from build123d import *

# Parameters (mm, degrees)
STOCK_BOX_1_START         = 83.223281248
STOCK_BOX_1_OUTLINE_W     = 122
STOCK_BOX_1_OUTLINE_H     = 102
STOCK_BOX_1_DEPTH         = 5
STOCK_BOX_1_START_2       = 80.223281248
STOCK_BOX_1_2_OUTLINE_W   = 118
STOCK_BOX_1_2_OUTLINE_H   = 98
STOCK_BOX_1_2_OUTLINE_W_2 = 114
STOCK_BOX_1_2_OUTLINE_H_2 = 94
STOCK_BOX_1_2_DEPTH       = 3
CUT_EXTRUDE2_REACH        = 168.26
SKETCH2_W                 = 19
SKETCH2_H                 = 3
SKETCH2_W_2               = 11
SKETCH3_W                 = 122
SKETCH3_H                 = 102
BOSS_EXTRUDE1_DEPTH       = 3
SKETCH4_W                 = 122
SKETCH4_H                 = 102
CUT_EXTRUDE3_DEPTH        = 3


# Read off the part's stored shape, not the designer's step: Stock-Box-1
with BuildPart() as part:
    # Stock-Box-1 outline → Stock-Box-1 (new body)
    with BuildSketch(Plane(origin=(0, 0, 0), x_dir=(1, 0, 0), z_dir=(0, 1, 0)).offset(STOCK_BOX_1_START)):
        with Locations((6.476673428, -22.886409736)):
            Rectangle(STOCK_BOX_1_OUTLINE_W, STOCK_BOX_1_OUTLINE_H)
    extrude(amount=STOCK_BOX_1_DEPTH)

    # Stock-Box-1 2 outline → Stock-Box-1 2 (add)
    with BuildSketch(Plane(origin=(0, 0, 0), x_dir=(1, 0, 0), z_dir=(0, 1, 0)).offset(STOCK_BOX_1_START_2)):
        with Locations((6.476673428, -22.886409736)):
            Rectangle(STOCK_BOX_1_2_OUTLINE_W, STOCK_BOX_1_2_OUTLINE_H)
        with Locations((6.476673428, -22.886409736)):
            Rectangle(STOCK_BOX_1_2_OUTLINE_W_2, STOCK_BOX_1_2_OUTLINE_H_2, mode=Mode.SUBTRACT)
    extrude(amount=STOCK_BOX_1_2_DEPTH)

    # Sketch2 → Cut-Extrude2 (cut, up to next)
    with BuildSketch(Plane.ZY.offset(52.523326572), mode=Mode.PRIVATE) as cut_extrude2_sk1:
        with Locations((-3.613590264, 81.723281248)):
            Rectangle(SKETCH2_W, SKETCH2_H)
    cut_extrude2_tool1 = extrude(cut_extrude2_sk1.sketch, amount=-CUT_EXTRUDE2_REACH, mode=Mode.PRIVATE) & part.part
    # Sketch2 → Cut-Extrude2 (cut, up to next)
    with BuildSketch(Plane.ZY.offset(52.523326572), mode=Mode.PRIVATE) as cut_extrude2_sk2:
        with Locations((21.386409736, 81.723281248)):
            Rectangle(SKETCH2_W_2, SKETCH2_H)
    cut_extrude2_tool2 = extrude(cut_extrude2_sk2.sketch, amount=-CUT_EXTRUDE2_REACH, mode=Mode.PRIVATE) & part.part
    add(cut_extrude2_tool1.solids().sort_by_distance((-52.523327, 81.723281, -3.61359))[0], mode=Mode.SUBTRACT)
    add(cut_extrude2_tool2.solids().sort_by_distance((-52.523327, 81.723281, 21.38641))[0], mode=Mode.SUBTRACT)

    # Sketch3 → Boss-Extrude1 (add)
    with BuildSketch(Plane(origin=(0, 88.223281248, 0), x_dir=(1, 0, 0), z_dir=(0, 1, 0))):
        with Locations((6.476673428, -22.886409736)):
            Rectangle(SKETCH3_W, SKETCH3_H)
    extrude(amount=-BOSS_EXTRUDE1_DEPTH)

    # Sketch4 → Cut-Extrude3 (cut)
    with BuildSketch(Plane(origin=(0, 88.223281248, 0), x_dir=(1, 0, 0), z_dir=(0, 1, 0))):
        with Locations((6.476673428, -22.886409736)):
            Rectangle(SKETCH4_W, SKETCH4_H)
    extrude(amount=-CUT_EXTRUDE3_DEPTH, mode=Mode.SUBTRACT)


solid = part.part
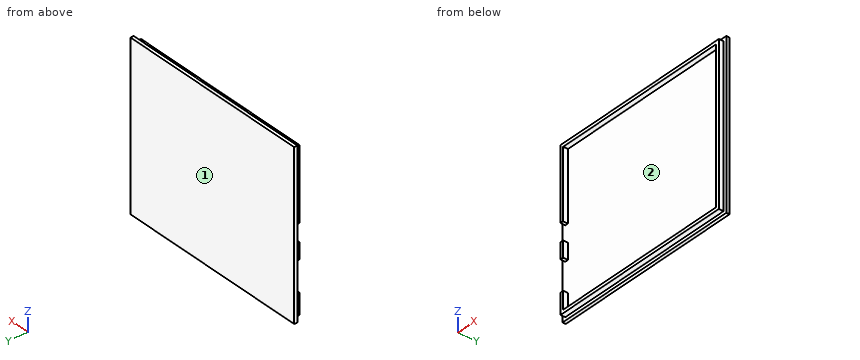
Verification items for the finished model (mm, model axes). Face numbers are marked on the shaded views. Coordinates: 2 decimals unless noted, no trailing zeros. Loops run counter-clockwise (first coordinate to the right, second up) from the corner with the lowest first, then second, coordinate; pieces in that order, holes last. Notation, with made-up numbers: (68, -6.5) -> (107, -6.5) arc R11 ccw to (107, 14.5) -> close; hole circle Ø3 at (37.25, 61). An arc over 180 degrees is marked (long way). Answer as a JSON object with one key per item and string values. Group by question number.
Item 1: Scan lines: probe 1 along X at (y, z) = (82.05, 9.5); probe 2 along Z at (x, y) = (-22.5, 81.2); probe 3 along Y at (x, z) = (50, 24.5). Record each from-to range of solid material in increasing order.
Item 2: Sectioned sample at C-C on z = 45. Record the boundary of the cut face in (x, y).
Item 3: Sectioned sample at A-A on y = 81.6. Record the boundary of the cut face in (x, z).
Item 4: Depth check by flat-ended pin: pin 1 (3 mm diameter, centred on x = 51.5, z = 34, fed in from -Y); pin 2 (0.9 mm diameter, centred on x = 12, y = 81.5, fed in from +Z); pin 3 (3 mm diameter, centred on x = 25.5, y = 81.5, fed in from -Z). Enter the tip coordinate at first touch or a pass-through.
Item 5: Sectioned sample at B-B on x = -15.5. Record the boundary of the cut face in (y, z), plus the area to 3 significant figures.
Item 6: Mould release check, pull along X, two halves, no side actions. Record for the marked faces 1 and 2: +X half, -X half, draft (parallel to the pull), parting line (faces both ways), or undercut.
Evaluation:
{
 "1": {"probe 1": "x = -52.52 to -50.52, 63.48 to 65.48", "probe 2": "z = -26.11 to -24.11, 69.89 to 71.89", "probe 3": "y = 83.22 to 85.22"},
 "2": {"outline": "(-54.52, 83.22) -> (-52.52, 83.22) -> (-52.52, 80.22) -> (-50.52, 80.22) -> (-50.52, 83.22) -> (63.48, 83.22) -> (63.48, 80.22) -> (65.48, 80.22) -> (65.48, 83.22) -> (67.48, 83.22) -> (67.48, 85.22) -> (-54.52, 85.22) -> close"},
 "3": {"outline": "(-52.52, -26.11) -> (65.48, -26.11) -> (65.48, 71.89) -> (-52.52, 71.89) -> (-52.52, 26.89) -> (-50.52, 26.89) -> (-50.52, 69.89) -> (63.48, 69.89) -> (63.48, -24.11) -> (-50.52, -24.11) -> (-50.52, -13.11) -> (-52.52, -13.11) -> close; (-52.52, 5.89) -> (-50.52, 5.89) -> (-50.52, 15.89) -> (-52.52, 15.89) -> close"},
 "4": {"pin 1": "stops at y = 83.22", "pin 2": "stops at z = 71.89", "pin 3": "stops at z = -26.11"},
 "5": {"outline": "(80.22, -26.11) -> (83.22, -26.11) -> (83.22, -28.11) -> (85.22, -28.11) -> (85.22, 73.89) -> (83.22, 73.89) -> (83.22, 71.89) -> (80.22, 71.89) -> (80.22, 69.89) -> (83.22, 69.89) -> (83.22, -24.11) -> (80.22, -24.11) -> close", "area": "216 mm²"},
 "6": {"face 1": "draft", "face 2": "undercut"}
}
